```python
from build123d import *

# Parameters (mm, degrees)
F0_W     = 200
F0_H     = 60
F1_DEPTH = 100
F3_DEPTH = 200


with BuildPart() as f1:
    # F0 (on Top) → F1 (new body)
    with BuildSketch(Plane.XY):
        Rectangle(F0_W, F0_H)
    extrude(amount=F1_DEPTH)

    # F2 (on face) → F3 (cut)
    with BuildSketch(Plane(origin=(-100, 0, 0), x_dir=(0, -1, 0), z_dir=(-1, 0, 0))):
        with BuildLine():
            Line((30, 100), (-20, 100))
            Line((-20, 100), (-20, 50))
            ThreePointArc((-20, 50), (-5.355339, 14.644661), (30, 0))
            Line((30, 0), (30, 100))
        make_face()
    extrude(amount=-F3_DEPTH, mode=Mode.SUBTRACT)


solid = f1.part
```
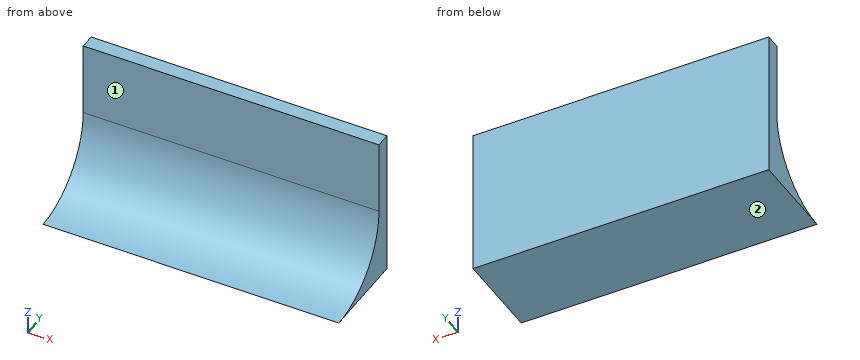
Could you check a few things on this model? Use its own coordinates, in mm. Face numbers are marked on the shaded views. A direction names the side the tool comes from. Coordinates: 2 decimals unless noted, no trailing zeros. Order: outer loops, then holes, each group sorted by start corner. A loop starts at its lowest first (then second) coordinate and runs counter-clockwise, first axis right, second up. Notation, with made-up numbers: M 24.5,-13.75 L 80.5,-13.75 A20 ccw 80.5,-2.75 Z; hole C 78.5,41.25 d8. An arc over 180 degrees is marked long. Use a Markdown table: item, result. Add a question column.
Q1. I want a section at C-C on y = -15.5. List the corners of the cut face in (x, z) for me, then the cut area to 3 significant figures.
Q2. If I drill on L1, parallel to Y at x = 26, z = 58; L2, parallel to Y at x = 20.5, z = 45; L3, parallel to Z at x = -25, y = 3.5, over which ranges is the centre line in solid material (lowest first)?
Q3. I'm going to push flat-ended pins straight in: pin 1 (25 mm diameter, centred on x = 10, z = 70.5, fed in from -Y); pin 2 (6 mm diameter, centred on x = 3.5, y = -20.5, fed in from +Z). Where does each tip first touch, or does it pass through?
Q4. I want a section at B-B on z = 60.5. List the corners of the cut face in (x, y) for me.
Q5. I want a section at A-A on x = -12.5. List the corners of the cut face in (y, z) for me, then the cut area to 3 significant figures.
Q6. Which directions (+Z, -Z, +X, -X, +Y, -Y) give clear straight access to the entire face, cutting with the end or side of a thin tool? Please do the marked faces 1 and 2.
Checked values:
| question | item | result |
|---|---|---|
| 1 | outline | M -100,0 L 100,0 L 100,2.15 L -100,2.15 Z |
| 1 | area | 430 mm² |
| 2 | L1 | 20 to 30 |
| 2 | L2 | 19.75 to 30 |
| 2 | L3 | 0 to 12.88 |
| 3 | pin 1 | y = 20 |
| 3 | pin 2 | z = 1.59 |
| 4 | outline | M -100,20 L 100,20 L 100,30 L -100,30 Z |
| 5 | outline | M -30,0 L 30,0 L 30,100 L 20,100 L 20,50 A50 cw Z |
| 5 | area | 1,540 mm² |
| 6 | face 1 | +Z, +X, -X, -Y |
| 6 | face 2 | -Z, +X, -X, +Y, -Y |
